Job drawing, mm, ordinate dimensions from the low corner. One solid piece. A direction names the side the tool comes from. Coordinates: 2 decimals unless noted, no trailing zeros. Order: outer loops, then holes, each group sorted by start corner. A loop starts at its lowest first (then second) coordinate and runs counter-clockwise, first axis right, second up. Notation, with made-up numbers: (-15.75, 38) - (13.25, 38) arc R8 cw to (13.25, 42) - close; hole circle Ø10 at (-21.75, -16.5). An arc over 180 degrees is marked (long way). Use a Markdown table: item, result. Add a question column.
1) Two-plate mould, pull along Y, no slides. Class the marked faces 1, 2, 3 and 4: +Y half, -Y half, draft (parallel to the pull), parting line (faces both ways), or undercut.
2) Saw through at B-B on x = 11.75. List the corners of the cut face in (y, z) (1 decimal).
3) Saw through at A-A on y = 9.25. List the corners of the cut face in (x, z).
4) Wall check: L1, parallel to Y at x = 9.5, z = 8.75 (1 decimal); L2, parallel to Z at x = 11.25, y = 20.25; L3, parallel to Y at x = 7, z = 11.5. Give the ranges that are in metal, low to high. Write a range as [from, to].
5) Drop flat-ended pins along their axis: P1, Ø12, axis at y = 3, z = 2, coming from the -X side; P2, Ø1, axis at x = 12.5, z = 13.5, coming from the -Y side; P3, Ø1.5, axis at x = 8.5, z = 17.5, coming from the +Y side. Give the stop position or say it passes through.
6) Tool access for the marked faces 5 and 6: list every direction of +Z, -Z, +X, -X, +Y, -Y with a clear straight run to the whole face (end or side of a thin tool).
7) Saw through at D-D on x = 3. List the corners of the cut face in (y, z) (1 decimal).
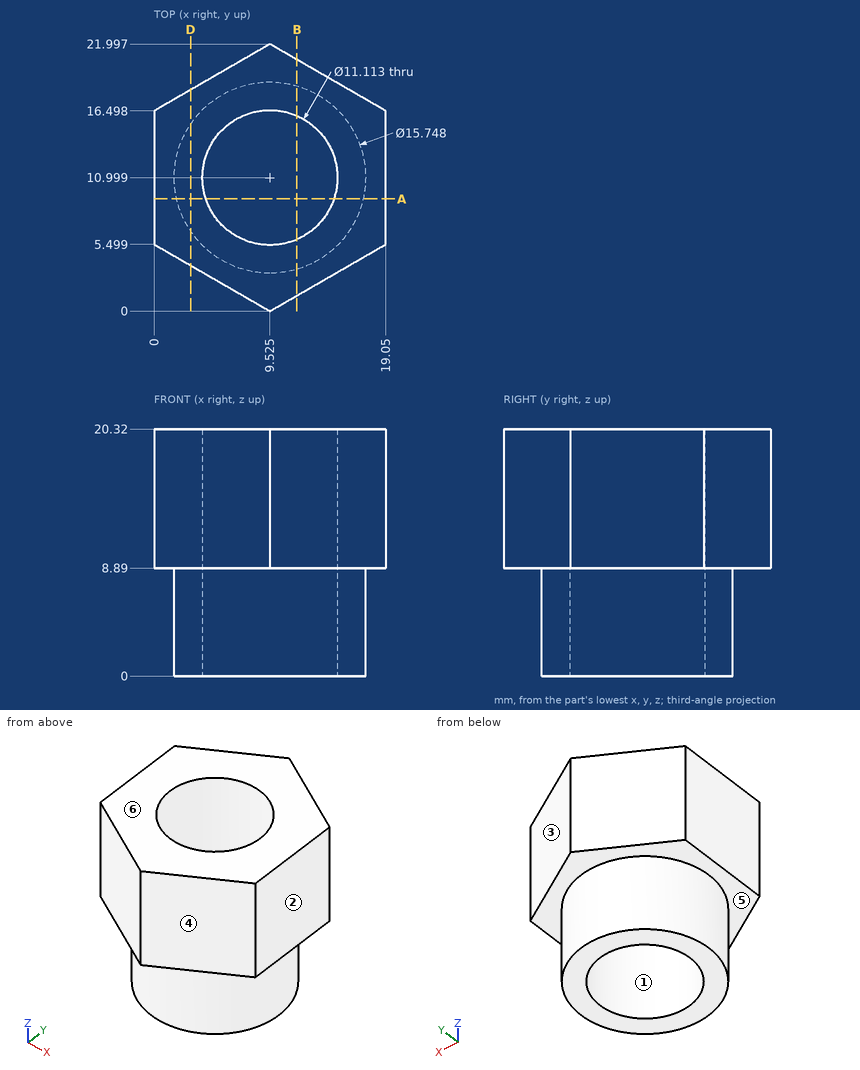
Results are:
| question | item | result |
|---|---|---|
| 1 | face 1 | undercut |
| 1 | face 2 | draft |
| 1 | face 3 | +Y half |
| 1 | face 4 | -Y half |
| 2 | outline | (1.3, 8.9) - (3.4, 8.9) - (3.4, 0) - (5.9, 0) - (5.9, 20.3) - (1.3, 20.3) - close; (16.1, 0) - (18.6, 0) - (18.6, 8.9) - (20.7, 8.9) - (20.7, 20.3) - (16.1, 20.3) - close |
| 3 | outline | (0, 8.89) - (1.85, 8.89) - (1.85, 0) - (4.25, 0) - (4.25, 20.32) - (0, 20.32) - close; (14.8, 0) - (17.2, 0) - (17.2, 8.89) - (19.05, 8.89) - (19.05, 20.32) - (14.8, 20.32) - close |
| 4 | L1 | [3.1, 5.4], [16.6, 18.9] |
| 4 | L2 | [8.89, 20.32] |
| 4 | L3 | [1.46, 6.05], [15.95, 20.54] |
| 5 | P1 | x = 1.91 |
| 5 | P2 | y = 1.43 |
| 5 | P3 | y = 21.84 |
| 6 | face 5 | -Z |
| 6 | face 6 | +Z, +X, -X, +Y, -Y |
| 7 | outline | (3.8, 8.9) - (6.6, 8.9) - (6.6, 0) - (15.4, 0) - (15.4, 8.9) - (18.2, 8.9) - (18.2, 20.3) - (3.8, 20.3) - close |
